from build123d import *

# Parameters (mm, degrees)
BOSS_EXTRUDE1_DEPTH = 3
SKETCH2_R           = 1
CUT_EXTRUDE1_DEPTH  = 43.679034666


with BuildPart() as part:
    # Sketch1 → Boss-Extrude1 (new body)
    with BuildSketch(Plane.XY):
        with BuildLine():
            Line((2.5, 40), (-2.5, 40))
            Line((-2.5, 40), (-2.5, -40))
            ThreePointArc((-2.5, -40), (0, -42.5), (2.5, -40))
            Line((2.5, -40), (2.5, 40))
        make_face()
    extrude(amount=BOSS_EXTRUDE1_DEPTH)

    # Sketch2 → Cut-Extrude1 (cut, through all)
    with BuildSketch(Plane.XY.offset(3)):
        with Locations((0, 35)):
            Circle(SKETCH2_R)
        with Locations((0.025500912, 20)):
            Circle(SKETCH2_R)
    extrude(amount=-CUT_EXTRUDE1_DEPTH, mode=Mode.SUBTRACT)


solid = part.part
Check sheet for the modelled part. Datum: model origin and axes. Units: mm. Round coordinates to 2 decimals unless told otherwise and drop trailing zeros. Order: outer loops, then holes, each group sorted by start corner. A loop starts at its lowest first (then second) coordinate and runs counter-clockwise, first axis right, second up.
Q1. Draft check along Y on faces 1 (the face through (0, 19, 2)), 2 (the face through (2.5, -1, 1)), 3 (the face through (-0.1, -42.5, 1.5)). Enter one of: pulls with the +Y half, pulls with the -Y half, needs draft (parallel to the pull), parting line crosses it, or undercut.
Filled sheet:
face 1: undercut
face 2: needs draft
face 3: pulls with the -Y half
Q2. Scan lines: L1, parallel to Y at x = 0, z = 2.35; L2, parallel to Y at x = 0.65, z = 2; L3, parallel to Y at x = -1.8, z = 1.1. Record each from-to range of solid material in increasing order.
Filled sheet:
L1: y = -42.5 to 19, 21 to 34, 36 to 40
L2: y = -42.41 to 19.22, 20.78 to 34.24, 35.76 to 40
L3: y = -41.73 to 40
Q3. Cross-section at C-C, the plane z = 1.4. Enter the section's corners in (x, y), plus the area to 3 significant figures.
Filled sheet:
outline: (-2.5, -40) arc R2.5 ccw to (2.5, -40) - (2.5, 40) - (-2.5, 40) - close; hole circle Ø2 at (0, 35); hole circle Ø2 at (0.03, 20)
area: 404 mm2
Q4. Cross-section at A-A, the plane y = 20. Enter the section's corners in (x, z).
Filled sheet:
outline: (-2.5, 0) - (-0.97, 0) - (-0.97, 3) - (-2.5, 3) - close; (1.03, 0) - (2.5, 0) - (2.5, 3) - (1.03, 3) - close
Q5. Cross-section at B-B, the plane x = 0. Enter the section's corners in (y, z), plus the area to 3 significant figures.
Filled sheet:
outline: (-42.5, 0) - (19, 0) - (19, 3) - (-42.5, 3) - close; (21, 0) - (34, 0) - (34, 3) - (21, 3) - close; (36, 0) - (40, 0) - (40, 3) - (36, 3) - close
area: 236 mm2
